The listing builds one solid part. Answer for the finished solid, in the listing's coordinates (mm). Face numbers are marked on the shaded views. A direction names the side the tool comes from. Round coordinates to 2 decimals unless told otherwise and drop trailing zeros. Order: outer loops, then holes, each group sorted by start corner. A loop starts at its lowest first (then second) coordinate and runs counter-clockwise, first axis right, second up. Notation, with made-up numbers: M -10.75,-11.5 L 45.25,-11.5 A28 cw 45.25,26.5 Z; hole C -34,-25.5 d5. An arc over 180 degrees is marked long. Write item = value, one per line. Start each with the question number.
(1) For a pull along Z with two mould halves and no side action, classify the marked faces 4, 5 and 6 as released by +Z, released by -Z, zero draft, split by the parting line, or undercut.
(2) Each of these flat-tipped pins is pushed along its axis until it touches: pin 1 (5 mm diameter, centred on x = 143.5, y = 25, fed in from -Z); pin 2 (1.5 mm diameter, centred on x = -98.5, y = 15.5, fed in from +Z); pin 3 (24 mm diameter, centred on x = 40.5, z = -139, fed in from +Y); pin 4 (24 mm diameter, centred on x = 214.5, z = 29, fed in from +Y). Where does it stop, or does it pass through?
(3) A cutting plane is placed at C-C, the plane y = 21. Determine the outline of the cut face in (x, z), and give its area (3 significant figures).
(4) A cutting plane is placed at A-A, the plane x = 144. Determine the outline of the cut face in (y, z), and give its area (3 significant figures).
(5) Straight lines are drawn through the part: probe 1 along X at (y, z) = (18, 28); probe 2 along Z at (x, y) = (95, 7.5); probe 3 along X at (y, z) = (5.5, -20.5). For each, find the intervals that lie inside material, in ascending order. Write a range as from..to.
(6) A cutting plane is placed at D-D, the plane z = 33. Determine the outline of the cut face in (x, y).
(7) Which of the six approach directions +Z, -Z, +X, -X, +Y, -Y give full straight-line access (tool end or side, diameter ignored) to the marked faces 1, 2 and 3?
(8) A cutting plane is placed at B-B, the plane z = -84.5. Determine the outline of the cut face in (x, y).
from build123d import *

# Parameters (mm, degrees)
SKETCH2_W            = 500
SKETCH2_H            = 200
BOSS_EXTRUDE1_DEPTH  = 37.5
CUT_EXTRUDE3_DEPTH   = 30
LPATTERN1_COUNT      = 2
LPATTERN1_PITCH      = 260
MIRROR1_COPY_1_DEPTH = 30
SKETCH7_W            = 460
SKETCH7_H            = 105
CUT_EXTRUDE4_DEPTH   = 160
FILLET1_R            = 10
FILLET2_R            = 10
FILLET3_R            = 10
FILLET4_R            = 10


with BuildPart() as part:
    # Sketch2 → Boss-Extrude1 (new body)
    with BuildSketch(Plane(origin=(0, 0, 0), x_dir=(1, 0, 0), z_dir=(0, 1, 0))):
        with Locations((0, 50)):
            Rectangle(SKETCH2_W, SKETCH2_H)
    extrude(amount=BOSS_EXTRUDE1_DEPTH)

    # Sketch5 → Cut-Extrude3 (cut)
    with BuildSketch(Plane(origin=(0, 0, -150), x_dir=(-1, 0, 0), z_dir=(0, 0, -1))):
        Polygon((24.5, 66.5), (54.5, 66.5), (54.5, 75), (205.5, 75), (205.5, 66.5), (235.5, 66.5), (235.5, 8.5), (205.5, 8.5), (205.5, 0), (54.5, 0), (54.5, 8.5), (24.5, 8.5), align=None)
    cut_extrude3 = extrude(amount=-CUT_EXTRUDE3_DEPTH, mode=Mode.SUBTRACT)

    # LPattern1: Cut-Extrude3 ×2
    with Locations(*[(i * LPATTERN1_PITCH, 0, 0) for i in range(1, LPATTERN1_COUNT)]):
        add(cut_extrude3, mode=Mode.SUBTRACT)

    # Mirror1: Cut-Extrude3 across plane
    add(cut_extrude3.mirror(Plane.XY.offset(-50)), mode=Mode.SUBTRACT)

    # Mirror1 copy 1 sketch → Mirror1 copy 1 (cut)
    with BuildSketch(Plane(origin=(260, 0, 50), x_dir=(-1, 0, 0), z_dir=(0, 0, 1))):
        Polygon((24.5, -66.5), (54.5, -66.5), (54.5, -75), (205.5, -75), (205.5, -66.5), (235.5, -66.5), (235.5, -8.5), (205.5, -8.5), (205.5, 0), (54.5, 0), (54.5, -8.5), (24.5, -8.5), align=None)
    extrude(amount=-MIRROR1_COPY_1_DEPTH, mode=Mode.SUBTRACT)

    # Sketch7 → Cut-Extrude4 (cut)
    with BuildSketch(Plane(origin=(0, 37.5, 0), x_dir=(1, 0, 0), z_dir=(0, 1, 0))):
        with Locations((0, 50)):
            Rectangle(SKETCH7_W, SKETCH7_H)
    extrude(amount=-CUT_EXTRUDE4_DEPTH, mode=Mode.SUBTRACT)

    # Fillet1
    fillet1_edges = [part.edges().sort_by_distance(p)[0] for p in [
        (-230, 18.75, -102.5),
    ]]
    fillet(fillet1_edges, radius=FILLET1_R)

    # Fillet2
    fillet2_edges = [part.edges().sort_by_distance(p)[0] for p in [
        (-230, 18.75, 2.5),
    ]]
    fillet(fillet2_edges, radius=FILLET2_R)

    # Fillet3
    fillet3_edges = [part.edges().sort_by_distance(p)[0] for p in [
        (230, 18.75, -102.5),
    ]]
    fillet(fillet3_edges, radius=FILLET3_R)

    # Fillet4
    fillet4_edges = [part.edges().sort_by_distance(p)[0] for p in [
        (230, 18.75, 2.5),
    ]]
    fillet(fillet4_edges, radius=FILLET4_R)


solid = part.part
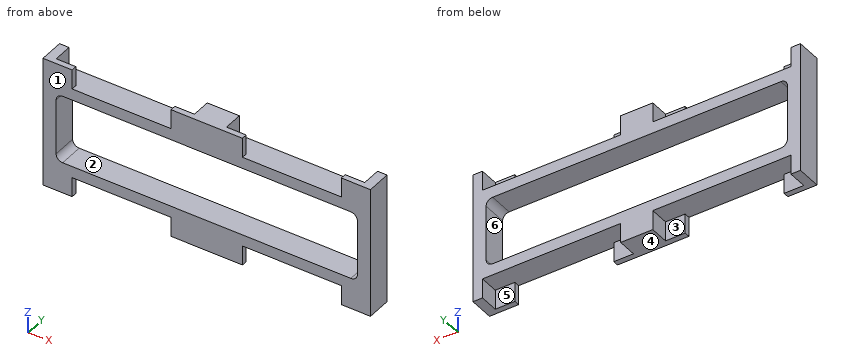
Reported:
q1.face_4 = released by -Z
q1.face_5 = zero draft
q1.face_6 = undercut
q2.pin_1 = -120
q2.pin_2 = 20
q2.pin_3 = 8.5
q2.pin_4 = 37.5
q3.outline = M -250,-150 L -235.5,-150 L -235.5,-120 L -24.5,-120 L -24.5,-150 L 24.5,-150 L 24.5,-120 L 235.5,-120 L 235.5,-150 L 250,-150 L 250,50 L 235.5,50 L 235.5,20 L 24.5,20 L 24.5,50 L -24.5,50 L -24.5,20 L -235.5,20 L -235.5,50 L -250,50 Z; hole M -230,-92.5 A10 ccw -220,-102.5 L 220,-102.5 A10 ccw 230,-92.5 L 230,-7.5 A10 ccw 220,2.5 L -220,2.5 A10 ccw -230,-7.5 Z
q3.area = 26,500 mm²
q4.outline = M 0,-120 L 37.5,-120 L 37.5,-102.5 L 0,-102.5 Z; M 0,2.5 L 37.5,2.5 L 37.5,20 L 0,20 Z
q4.area = 1,310 mm²
q5.probe_1 = -250..-235.5, -24.5..24.5, 235.5..250
q5.probe_2 = -120..-102.5, 2.5..20
q5.probe_3 = -250..-230, 230..250
q6.outline = M -250,0 L -205.5,0 L -205.5,8.5 L -235.5,8.5 L -235.5,37.5 L -250,37.5 Z; M -54.5,0 L 54.5,0 L 54.5,8.5 L 24.5,8.5 L 24.5,37.5 L -24.5,37.5 L -24.5,8.5 L -54.5,8.5 Z; M 205.5,0 L 250,0 L 250,37.5 L 235.5,37.5 L 235.5,8.5 L 205.5,8.5 Z
q7.face_1 = +Z, -Z, +X, -X, -Y
q7.face_2 = +Y, -Y
q7.face_3 = -Z, +Y
q8.outline = M -250,0 L -230,0 L -230,37.5 L -250,37.5 Z; M 230,0 L 250,0 L 250,37.5 L 230,37.5 Z
